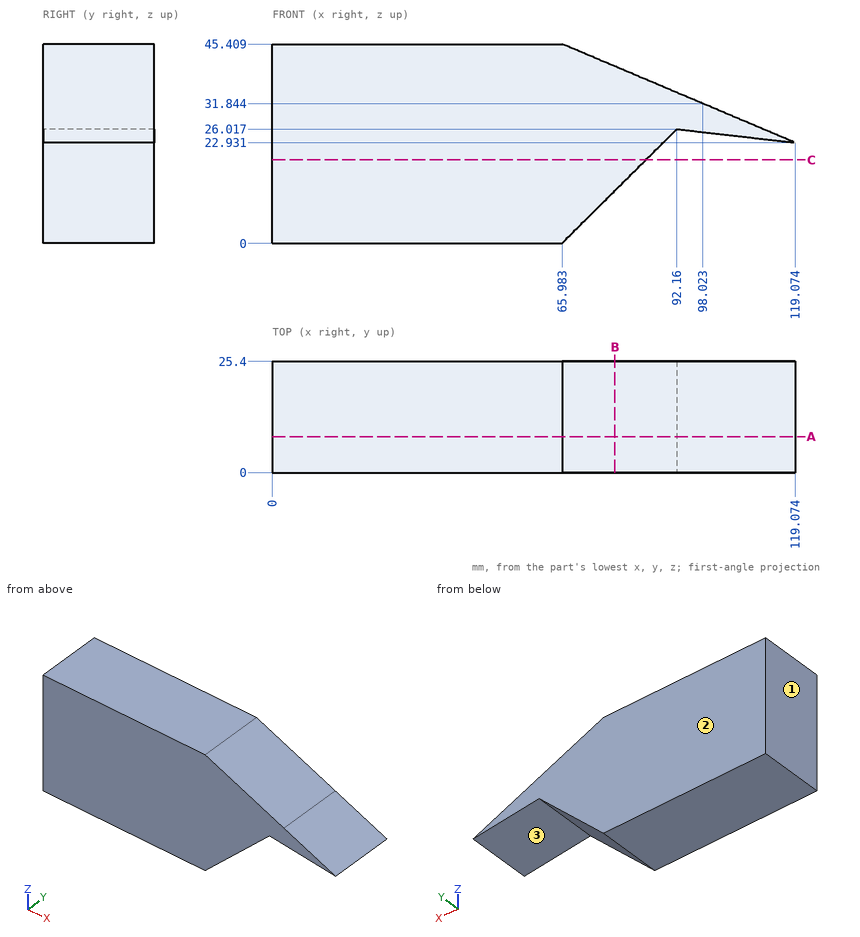
For this review, use the dimensioned drawing (mm, ordinates from the lowest corner) and the shaded views. Round coordinates to 2 decimals unless told otherwise and drop trailing zeros. Order: outer loops, then holes, each group sorted by start corner. A loop starts at its lowest first (then second) coordinate and runs counter-clockwise, first axis right, second up. Notation, with made-up numbers: (-28, 58.5) -> (23, 58.5) arc R17 cw to (23, 67.5) -> close; hole circle Ø11 at (-16, 17.25). An arc over 180 degrees is marked (long way). One line per item, written item: value. Start each with the question number.
Q1. Take a section at B-B (x = 78). Write out the cut boundary in (y, z), and give its area (3 significant figures).
Q2. Wall thickness on line 1 (X direction, y = 19.5, z = 16); line 2 (X direction, y = 23.75, z = 7) (1 decimal); line 3 (Z direction, x = 82.5, y = 4.5) (1 decimal): over which ranges is each line inside the solid? List them lowest first.
Q3. Take a section at A-A (y = 8.25). Write out the cut boundary in (x, z) (1 decimal), and give its area (3 significant figures).
Q4. Clearance check with flat-ended pins moving along their axes: pin 1 Ø12 at (x, z) = (103.5, 40.5) entering from +Y; pin 2 Ø2 at (x, y) = (70, 10) entering from -Z; pin 3 Ø1 at (x, y) = (68.5, 10) entering from +Z (1 decimal); pin 4 Ø10 at (y, z) = (2.5, 8) entering from +X. State where each tip first meets the part, or that it passes through.
Q5. Take a section at C-C (z = 19). Write out the cut boundary in (x, y), and give its area (3 significant figures).
Q6. Mouldability with a two-part tool opening along X and no side actions: class the marked faces 1, 2 and 3 as released by +X, released by -X, zero draft, split by the parting line, or undercut.
Reported:
1. outline: (0, 11.94) -> (25.4, 11.94) -> (25.4, 40.32) -> (0, 40.32) -> close
1. area: 721 mm2
2. line 1: x = 0 to 82.08
2. line 2: x = 0 to 73
2. line 3: z = 16.4 to 38.4
3. outline: (0, 0) -> (66, 0) -> (92.2, 26) -> (119.1, 22.9) -> (66, 45.4) -> (0, 45.4) -> close
3. area: 3,810 mm2
4. pin 1: passes through
4. pin 2: stops at z = 3
4. pin 3: stops at z = 44.6
4. pin 4: stops at x = 79.06
5. outline: (0, 0) -> (85.1, 0) -> (85.1, 25.4) -> (0, 25.4) -> close
5. area: 2,160 mm2
6. face 1: released by -X
6. face 2: zero draft
6. face 3: undercut
